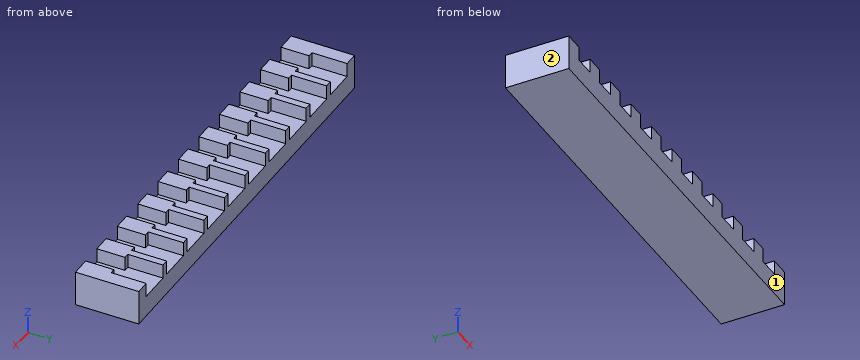
Autodesk Fusion 360 part; units mm, degrees
sketch "Sketch1" plane through (0, 0, 0) normal (0, 0, 1) x (1, 0, 0)
  line L0 (0, 57.15) -> (0, 0)
  line L1 (12.7, 57.15) -> (41.275, 57.15)
  line L2 (41.275, 57.15) -> (41.275, 25.4)
  line L3 (41.275, 25.4) -> (12.7, 25.4)
  line L4 (12.7, 25.4) -> (12.7, 57.15)
  line L5 (26.9875, 25.4) -> (26.9875, 0) construction
  line L6 (17.4625, 25.4) -> (17.4625, 0)
  line L7 (36.5125, 25.4) -> (36.5125, 0)
  line L8 (17.4625, 0) -> (36.5125, 0)
  line L9 (52.3875, 25.4) -> (52.3875, 0)
  line L10 (47.625, 57.15) -> (76.2, 57.15)
  line L11 (61.9125, 25.4) -> (61.9125, 0) construction
  line L12 (47.625, 25.4) -> (47.625, 57.15)
  line L13 (76.2, 25.4) -> (47.625, 25.4)
  line L14 (76.2, 57.15) -> (76.2, 25.4)
  line L15 (71.4375, 25.4) -> (71.4375, 0)
  line L16 (52.3875, 0) -> (71.4375, 0)
  line L17 (87.3125, 25.4) -> (87.3125, 0)
  line L18 (82.55, 57.15) -> (111.125, 57.15)
  line L19 (96.8375, 25.4) -> (96.8375, 0) construction
  line L20 (82.55, 25.4) -> (82.55, 57.15)
  line L21 (111.125, 25.4) -> (82.55, 25.4)
  line L22 (111.125, 57.15) -> (111.125, 25.4)
  line L23 (106.3625, 25.4) -> (106.3625, 0)
  line L24 (87.3125, 0) -> (106.3625, 0)
  line L25 (122.2375, 25.4) -> (122.2375, 0)
  line L26 (117.475, 57.15) -> (146.05, 57.15)
  line L27 (131.7625, 25.4) -> (131.7625, 0) construction
  line L28 (117.475, 25.4) -> (117.475, 57.15)
  line L29 (146.05, 25.4) -> (117.475, 25.4)
  line L30 (146.05, 57.15) -> (146.05, 25.4)
  line L31 (141.2875, 25.4) -> (141.2875, 0)
  line L32 (122.2375, 0) -> (141.2875, 0)
  line L33 (368.3, 57.15) -> (368.3, 0)
  line L34 (368.3, 0) -> (0, 0)
  line L35 (368.3, 57.15) -> (0, 57.15)
  line L36 (176.2125, 25.4) -> (176.2125, 0)
  line L37 (152.4, 57.15) -> (180.975, 57.15)
  line L38 (166.6875, 25.4) -> (166.6875, 0) construction
  line L39 (157.1625, 25.4) -> (157.1625, 0)
  line L40 (180.975, 25.4) -> (152.4, 25.4)
  line L41 (157.1625, 0) -> (176.2125, 0)
  line L42 (180.975, 57.15) -> (180.975, 25.4)
  line L43 (152.4, 25.4) -> (152.4, 57.15)
  line L44 (211.1375, 25.4) -> (211.1375, 0)
  line L45 (187.325, 57.15) -> (215.9, 57.15)
  line L46 (201.6125, 25.4) -> (201.6125, 0) construction
  line L47 (192.0875, 25.4) -> (192.0875, 0)
  line L48 (215.9, 25.4) -> (187.325, 25.4)
  line L49 (192.0875, 0) -> (211.1375, 0)
  line L50 (215.9, 57.15) -> (215.9, 25.4)
  line L51 (187.325, 25.4) -> (187.325, 57.15)
  line L52 (246.0625, 25.4) -> (246.0625, 0)
  line L53 (227.0125, 0) -> (246.0625, 0)
  line L54 (222.25, 57.15) -> (250.825, 57.15)
  line L55 (222.25, 25.4) -> (222.25, 57.15)
  line L56 (227.0125, 25.4) -> (227.0125, 0)
  line L57 (236.5375, 25.4) -> (236.5375, 0) construction
  line L58 (250.825, 25.4) -> (222.25, 25.4)
  line L59 (250.825, 57.15) -> (250.825, 25.4)
  line L60 (280.9875, 25.4) -> (280.9875, 0)
  line L61 (261.9375, 0) -> (280.9875, 0)
  line L62 (257.175, 57.15) -> (285.75, 57.15)
  line L63 (257.175, 25.4) -> (257.175, 57.15)
  line L64 (261.9375, 25.4) -> (261.9375, 0)
  line L65 (271.4625, 25.4) -> (271.4625, 0) construction
  line L66 (285.75, 25.4) -> (257.175, 25.4)
  line L67 (285.75, 57.15) -> (285.75, 25.4)
  line L68 (315.9125, 25.4) -> (315.9125, 0)
  line L69 (296.8625, 0) -> (315.9125, 0)
  line L70 (292.1, 57.15) -> (320.675, 57.15)
  line L71 (292.1, 25.4) -> (292.1, 57.15)
  line L72 (296.8625, 25.4) -> (296.8625, 0)
  line L73 (306.3875, 25.4) -> (306.3875, 0) construction
  line L74 (320.675, 25.4) -> (292.1, 25.4)
  line L75 (320.675, 57.15) -> (320.675, 25.4)
  line L76 (350.8375, 25.4) -> (350.8375, 0)
  line L77 (331.7875, 0) -> (350.8375, 0)
  line L78 (327.025, 57.15) -> (355.6, 57.15)
  line L79 (327.025, 25.4) -> (327.025, 57.15)
  line L80 (331.7875, 25.4) -> (331.7875, 0)
  line L81 (341.3125, 25.4) -> (341.3125, 0) construction
  line L82 (355.6, 25.4) -> (327.025, 25.4)
  line L83 (355.6, 57.15) -> (355.6, 25.4)
  dimension "d2" = 57.15
  dimension "d4" = 28.575
  dimension "d6" = 9.525
  dimension "d7" = 9.525
  dimension "d39" = 31.75
  dimension "d40" = 28.575
  dimension "d41" = 9.525
  dimension "d42" = 9.525
  dimension "d43" = 31.75
  dimension "d44" = 28.575
  dimension "d45" = 9.525
  dimension "d46" = 9.525
  dimension "d47" = 31.75
  dimension "d48" = 28.575
  dimension "d49" = 9.525
  dimension "d50" = 9.525
  dimension "d51" = 31.75
  dimension "d52" = 6.35
  dimension "d53" = 6.35
  dimension "d54" = 6.35
  dimension "d56" = 28.575
  dimension "d57" = 9.525
  dimension "d58" = 9.525
  dimension "d59" = 31.75
  dimension "d60" = 28.575
  dimension "d61" = 9.525
  dimension "d62" = 9.525
  dimension "d63" = 31.75
  dimension "d64" = 6.35
  dimension "d65" = 6.35
  dimension "d77" = 12.7
  dimension "d78" = 28.575
  dimension "d79" = 9.525
  dimension "d80" = 9.525
  dimension "d81" = 31.75
  dimension "d82" = 28.575
  dimension "d83" = 9.525
  dimension "d84" = 9.525
  dimension "d85" = 31.75
  dimension "d86" = 6.35
  dimension "d87" = 6.35
  dimension "d89" = 28.575
  dimension "d90" = 9.525
  dimension "d91" = 9.525
  dimension "d92" = 31.75
  dimension "d93" = 28.575
  dimension "d94" = 9.525
  dimension "d95" = 9.525
  dimension "d96" = 31.75
  dimension "d97" = 12.7
  dimension "d98" = 6.35
  dimension "d99" = 6.35
extrude "Extrude8" add sketch "Sketch1" against normal blind 31.75
extrude "Extrude9" cut sketch "Sketch1" against normal blind 12.7 contours L1 L2 L3 L4 L35 | L3 L6 L7 L8 L34 | L10 L12 L13 L14 L35 | L9 L13 L15 L16 L34 | L18 L20 L21 L22 L35 | L17 L21 L23 L24 L34 | L26 L28 L29 L30 L35 | L25 L29 L31 L32 L34 | L35 L37 L40 L42 L43 | L34 L36 L39 L40 L41 | L35 L45 L48 L50 L51 | L34 L44 L47 L48 L49 | L35 L54 L55 L58 L59 | L34 L52 L53 L56 L58 | L35 L62 L63 L66 L67 | L34 L60 L61 L64 L66 | L35 L70 L71 L74 L75 | L34 L68 L69 L72 L74 | L35 L78 L79 L82 L83 | L34 L76 L77 L80 L82
Geometry check sheet. Reference: the model listing, model coordinates, mm. Face numbers are marked on the shaded views. Round coordinates to 2 decimals unless told otherwise and drop trailing zeros. Loops run counter-clockwise (first coordinate to the right, second up) from the corner with the lowest first, then second, coordinate; pieces in that order, holes last. Notation, with made-up numbers: (36, -4.5) - (54, -4.5) arc R26 ccw to (54, 32.5) - close; hole circle Ø8 at (7.25, -6). An arc over 180 degrees is marked (long way). Write item = value, one per line. Start each with the question number.
1. Section check B-B on x = 24. Enter the section's corners in (y, z), then the cut area to 3 significant figures.
2. Section check A-A on z = -3. Give the number of separate pieces and of enclosed holes in the cut face, then the cut area to 3 significant figures.
3. Mould release check, pull along Y, two halves, no side actions. Record for the marked faces 1 and 2: released by +Y, released by -Y, zero draft, split by the parting line, or undercut.
4. Thickness scan on line 1 (Z direction, x = 230, y = 14). Record the ranges inside material, lowest first.
5. Depth check by flat-ended pin: pin 1 (2.5 mm diameter, centred on x = 295, z = -6.5, fed in from +Y); pin 2 (8.5 mm diameter, centred on x = 338, y = 26.5, fed in from +Z). Enter the tip coordinate at first touch or a pass-through.
Working result:
q1.outline = (0, -31.75) - (57.15, -31.75) - (57.15, -12.7) - (0, -12.7) - close
q1.area = 1,090 mm^2
q2.separate_pieces = 11
q2.enclosed_holes = 0
q2.area = 7,140 mm^2
q3.face_1 = released by -Y
q3.face_2 = zero draft
q4.line_1 = -31.75 to -12.7
q5.pin_1 = 25.4
q5.pin_2 = -12.7
